Check sheet for the modelled part. Datum: model origin and axes. Units: mm. A direction names the side the tool comes from. Round coordinates to 2 decimals unless told otherwise and drop trailing zeros. One line per item, written item: value.
from build123d import *

# Parameters (mm, degrees)
SKETCH_1_W          = 25
SKETCH_1_H          = 50
EXTRUDE_1_DEPTH     = 550
SKETCH_2_R          = 4
CUT_EXTRUDE_1_DEPTH = 10
CUT_EXTRUDE_START   = -10
SKETCH_3_R          = 4
CUT_EXTRUDE_2_DEPTH = 10
SKETCH_4_W          = 25
SKETCH_4_H          = 50
CUT_EXTRUDE_3_DEPTH = 50


with BuildPart() as part:
    # Эскиз1 → Бобышка-Вытянуть1 (new body)
    with BuildSketch(Plane(origin=(0, 0, 0), x_dir=(1, 0, 0), z_dir=(0, 1, 0))):
        Rectangle(SKETCH_1_W, SKETCH_1_H)
    extrude(amount=EXTRUDE_1_DEPTH)

    # Эскиз2 → Вырез-Вытянуть1 (cut)
    with BuildSketch(Plane(origin=(0, 550, 0), x_dir=(1, 0, 0), z_dir=(0, 1, 0))):
        with Locations(Location((0, 0, 0), (0, 0, 270))):
            Circle(SKETCH_2_R)
    extrude(amount=-CUT_EXTRUDE_1_DEPTH, mode=Mode.SUBTRACT)

    # Эскиз3 → Вырез-Вытянуть2 (cut)
    with BuildSketch(Plane.XZ.offset(CUT_EXTRUDE_START)):
        with Locations(Location((0, 0, 0), (0, 0, 90))):
            Circle(SKETCH_3_R)
    extrude(amount=CUT_EXTRUDE_2_DEPTH, mode=Mode.SUBTRACT)

    # Эскиз4 → Вырез-Вытянуть3 (cut)
    with BuildSketch(Plane(origin=(0, 550, 0), x_dir=(1, 0, 0), z_dir=(0, 1, 0))):
        Rectangle(SKETCH_4_W, SKETCH_4_H)
    extrude(amount=-CUT_EXTRUDE_3_DEPTH, mode=Mode.SUBTRACT)


solid = part.part
Item 1: Mould release check, pull along X, two halves, no side actions. Record for faces 1 (the flat face through (12.5, 246, 0)), 2 (the flat face through (0, 246, -25)), 3 (the flat face through (0, 10, 0)): pulls with the +X half, pulls with the -X half, needs draft (parallel to the pull), parting line crosses it, or undercut.
Answer:
face 1: pulls with the +X half
face 2: needs draft
face 3: undercut
Item 2: Tool access check on faces 4 (the cylindrical face through (3.905, 5.07, -0.867)), 5 (the flat face through (-12.5, 246, 0)). Record the directions out of +Z, -Z, +X, -X, +Y, -Y that give a thin tool (end or side, any length) a straight path to the whole face; none if there is none.
Answer:
face 4: -Y
face 5: +Z, -Z, -X, +Y, -Y
Item 3: Thickness scan on line 1 (X direction, y = 5, z = 0); line 2 (Y direction, x = -2.25, z = 1.5). Record the ranges inside material, lowest first.
Answer:
line 1: x = -12.5 to -4, 4 to 12.5
line 2: y = 10 to 500
